Source: CAD feature listing. Evaluate the final solid. Frame: model axes, mm. Face numbers are marked on the shaded views. A direction names the side the tool comes from. Coordinates: 2 decimals unless noted, no trailing zeros. Write each loop counter-clockwise with the first axis right and the second up, starting at its lowest first coordinate (ties: lowest second). Pieces come first, ordered by that corner, then holes. Notation, with made-up numbers: M 15,13.5 L 50,13.5 A12 ccw 50,21.5 Z; hole C 45,78 d4. An arc over 180 degrees is marked long. One line per item, written item: value. Start each with the question number.
Item 1: Cut plane A-A, the plane z = 50. Output: boundary loops of the cut face in (x, y).
Item 2: Ray query, L1, parallel to Y at x = -24.85, z = 28.5; L2, parallel to X at y = 27, z = 50; L3, parallel to Z at x = 24, y = -10. Return the intervals inside material, ascending. Write a range as from..to.
Item 3: Cut plane B-B, the plane y = -23. Output: boundary loops of the cut face in (x, z).
Item 4: Set-up query: the marked faces 5, 6 and 7. Return all of +Z, -Z, +X, -X, +Y, -Y with unobstructed straight access to the full face (end or side cutting, diameter ignored); none if empty.
Item 5: Cut plane C-C, the plane z = 23. Output: boundary loops of the cut face in (x, y).
Item 6: Pin query (flat end, axial travel): P1, Ø3, axis at x = -16.5, z = 50.5, coming from the -Y side; P2, Ø4, axis at x = -24.85, y = 5, coming from the +Z side; P3, Ø3, axis at x = 25.5, y = -6, coming from the +Z side. Return the tip coordinate at first contact, or that it passes through.
Item 7: Mould query, pull axis Z, two halves, no side actions, for the marked faces 1, 2, 3 and 4. Classes: released by +Z, released by -Z, zero draft, split by the parting line, or undercut.
Item 8: Cut plane D-D, the plane x = 1. Output: boundary loops of the cut face in (y, z).
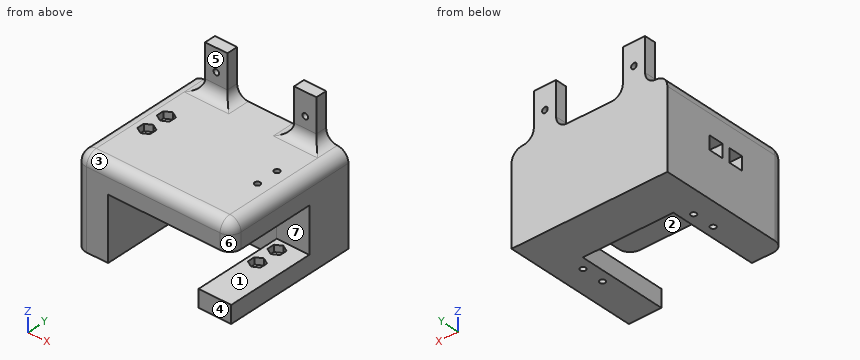
```python
from build123d import *

# Parameters (mm, degrees)
SKETCH_2_W           = 70
SKETCH_2_H           = 60
EXTRUDE_2_DEPTH      = 40
SKETCH_3_W           = 40.7
SKETCH_3_H           = 20.5
CUT_EXTRUDE_1_DEPTH  = 28
SKETCH_4_W           = 14.65
SKETCH_4_H           = 20.5
EXTRUDE_3_DEPTH      = 28
SKETCH_8_W           = 10
SKETCH_8_H           = 5
EXTRUDE_5_DEPTH      = 60
SKETCH_15_W          = 40.7
SKETCH_15_H          = 40.25
CUT_EXTRUDE_6_DEPTH  = 28
SKETCH_16_W          = 14.65
SKETCH_16_H          = 20.204149113
CUT_EXTRUDE_7_DEPTH  = 40
M3X0_5_1_D           = 2.5
FILLET_1_R           = 5
FILLET_2_R           = 5
FILLET_3_R           = 5
M3X0_5_2_D           = 2.5
CUT_EXTRUDE_8_DEPTH  = 3
CUT_EXTRUDE_9_DEPTH  = 3
CUT_EXTRUDE_10_DEPTH = 6


# Some blends are built 0.0001 mm under size
with BuildPart() as part:
    # ｽｹｯﾁ2 → ﾎﾞｽ - 押し出し2 (new body)
    with BuildSketch(Plane.XY):
        Rectangle(SKETCH_2_W, SKETCH_2_H)
    extrude(amount=EXTRUDE_2_DEPTH)

    # ｽｹｯﾁ3 → ｶｯﾄ - 押し出し1 (cut)
    with BuildSketch(Plane.XY):
        Rectangle(SKETCH_3_W, SKETCH_3_H)
    extrude(amount=CUT_EXTRUDE_1_DEPTH, mode=Mode.SUBTRACT)

    # ｽｹｯﾁ4 → ﾎﾞｽ - 押し出し3 (add)
    with BuildSketch(Plane.XY):
        with Locations((27.675, 0)):
            Rectangle(SKETCH_4_W, SKETCH_4_H)
    extrude(amount=EXTRUDE_3_DEPTH)

    # ｽｹｯﾁ8 → ﾎﾞｽ - 押し出し5 (add)
    with BuildSketch(Plane.XY):
        with Locations((-20, 27.5)):
            Rectangle(SKETCH_8_W, SKETCH_8_H)
        with Locations((20, 27.5)):
            Rectangle(SKETCH_8_W, SKETCH_8_H)
    extrude(amount=EXTRUDE_5_DEPTH)

    # ｽｹｯﾁ15 → ｶｯﾄ - 押し出し6 (cut)
    with BuildSketch(Plane.XY):
        with Locations((0, -9.875)):
            Rectangle(SKETCH_15_W, SKETCH_15_H)
    extrude(amount=CUT_EXTRUDE_6_DEPTH, mode=Mode.SUBTRACT)

    # ｽｹｯﾁ16 → ｶｯﾄ - 押し出し7 (cut)
    with BuildSketch(Plane(origin=(0, -30, 0), x_dir=(-1, 0, 0), z_dir=(0, -1, 0))):
        with Locations((-27.675, -17.897925444)):
            Rectangle(SKETCH_16_W, SKETCH_16_H)
    extrude(amount=-CUT_EXTRUDE_7_DEPTH, mode=Mode.SUBTRACT)

    # M3x0.5 ねじ穴1 (through all)
    with Locations(Plane(origin=(0, 30, 0), x_dir=(1, 0, 0), z_dir=(0, 1, 0))):
        with Locations((-20, -50), (20, -50)):
            Hole(M3X0_5_1_D / 2)

    # ﾌｨﾚｯﾄ1
    fillet_1_edges = [part.edges().sort_by_distance(p)[0] for p in [
        (-15, 27.5, 40),
        (-20, 25, 40),
        (-25, 27.5, 40),
        (20, 25, 40),
        (15, 27.5, 40),
        (25, 27.5, 40),
    ]]
    fillet(fillet_1_edges, radius=FILLET_1_R)

    # ﾌｨﾚｯﾄ2
    fillet_2_edges = [part.edges().sort_by_distance(p)[0] for p in [
        (35, 0, 40),
        (35, -30, 34),
        (0, -30, 40),
        (-35, 0, 40),
    ]]
    fillet(fillet_2_edges, radius=FILLET_2_R - 0.0001)  # a hair under: the kernel refuses the full size

    # ﾌｨﾚｯﾄ3
    # the kernel refuses this fillet: 5 mm, written as the material it takes off along each edge
    with BuildSketch(Plane(origin=(-30, -25, 40), x_dir=(-1, 0, 0), z_dir=(0, 1, 0))) as fillet_3_piece_1:
        with BuildLine():
            CenterArc((0.0001, -4.9999), 4.9999, 0, 90)
            Line((5, -4.9999), (5, 0))
            Line((5, 0), (0.0001, 0))
        make_face()
    revolve(axis=Axis((-30, -25, 40), (0, 0, 1)), revolution_arc=90, mode=Mode.SUBTRACT)
    with BuildSketch(Plane(origin=(-35, -30, -12.5), x_dir=(0, 1, 0), z_dir=(0, 0, 1))) as fillet_3_piece_2:
        with BuildLine():
            CenterArc((FILLET_3_R, -FILLET_3_R), FILLET_3_R, 90, 90)
            Line((0, -FILLET_3_R), (0, 0))
            Line((0, 0), (FILLET_3_R, 0))
        make_face()
    extrude(amount=52.5, mode=Mode.SUBTRACT)

    # M3x0.5 ねじ穴2 (through all)
    with Locations(Plane(origin=(0, 0, 0), x_dir=(-1, 0, 0), z_dir=(0, 0, -1))):
        with Locations((24.85, 5), (24.85, -5)):
            m3x0_5_2 = Hole(M3X0_5_2_D / 2)

    # ﾐﾗｰ1: M3x0.5 ねじ穴2 across plane
    add(m3x0_5_2.mirror(Plane(origin=(0, 0, 0), x_dir=(0, 0, 1), z_dir=(1, 0, 0))), mode=Mode.SUBTRACT)

    # ｽｹｯﾁ17 → ｶｯﾄ - 押し出し8 (cut)
    with BuildSketch(Plane.XY.offset(40)):
        Polygon((-24.85, 8.290896534), (-27.7, 6.645448267), (-27.7, 3.354551733), (-24.85, 1.709103466), (-22, 3.354551733), (-22, 6.645448267), align=None)
        Polygon((-22, -6.645448267), (-22, -3.354551733), (-24.85, -1.709103466), (-27.7, -3.354551733), (-27.7, -6.645448267), (-24.85, -8.290896534), align=None)
    extrude(amount=-CUT_EXTRUDE_8_DEPTH, mode=Mode.SUBTRACT)

    # ｽｹｯﾁ18 → ｶｯﾄ - 押し出し9 (cut)
    with BuildSketch(Plane.XY.offset(7.795850887)):
        Polygon((27.7, 3.354551733), (27.7, 6.645448267), (24.85, 8.290896534), (22, 6.645448267), (22, 3.354551733), (24.85, 1.709103466), align=None)
        Polygon((27.7, -6.645448267), (27.7, -3.354551733), (24.85, -1.709103466), (22, -3.354551733), (22, -6.645448267), (24.85, -8.290896534), align=None)
    extrude(amount=-CUT_EXTRUDE_9_DEPTH, mode=Mode.SUBTRACT)

    # ｽｹｯﾁ19 → ｶｯﾄ - 押し出し10 (cut)
    with BuildSketch(Plane(origin=(0, 0, 20), x_dir=(-1, 0, 0), z_dir=(0, 0, -1))):
        Polygon((35, 1.709103466), (35, 8.290896534), (24.85, 8.290896534), (27.7, 6.645448267), (27.7, 3.354551733), (24.85, 1.709103466), align=None)
        Polygon((22, 6.645448267), (22, 3.354551733), (24.85, 1.709103466), (27.7, 3.354551733), (27.7, 6.645448267), (24.85, 8.290896534), align=None)
        Polygon((22, -6.645448267), (24.85, -8.290896534), (27.7, -6.645448267), (27.7, -3.354551733), (24.85, -1.709103466), (22, -3.354551733), align=None)
        Polygon((35, -8.290896534), (24.85, -8.290896534), (27.7, -6.645448267), (27.7, -3.354551733), (24.85, -1.709103466), (35, -1.709103466), align=None)
    extrude(amount=-CUT_EXTRUDE_10_DEPTH, mode=Mode.SUBTRACT)


solid = part.part
```
From the geometry:
1. outline: M -25,25 L -21.25,25 L -21.25,30 L -25,30 Z; M -18.75,25 L -15,25 L -15,30 L -18.75,30 Z; M 15,25 L 18.75,25 L 18.75,30 L 15,30 Z; M 21.25,25 L 25,25 L 25,30 L 21.25,30 Z
2. L1: y = -30..-6.25, -3.75..3.75, 6.25..30
2. L2: x = -25..-21.25, -18.75..-15, 15..18.75, 21.25..25
2. L3: z = 0..7.8, 28..40
3. outline: M -35,0 L -20.35,0 L -20.35,28 L 35,28 L 35,35 A5 ccw 30,40 L -30,40 A5 ccw -35,35 Z; M 20.35,0 L 35,0 L 35,7.8 L 20.35,7.8 Z
4. face 5: +Z, +X, -X, -Y
4. face 6: +Z, +X, -Y
4. face 7: +X, -Y
5. outline: M -35,-25 A5 ccw -30,-30 L -20.35,-30 L -20.35,10.25 L 20.35,10.25 L 20.35,10 L 35,10 L 35,30 L -35,30 L -35,8.29 L -24.85,8.29 L -22,6.65 L -22,3.35 L -24.85,1.71 L -35,1.71 L -35,-1.71 L -24.85,-1.71 L -22,-3.35 L -22,-6.65 L -24.85,-8.29 L -35,-8.29 Z
6. P1: stops at y = 25
6. P2: stops at z = 37
6. P3: stops at z = 40
7. face 1: undercut
7. face 2: undercut
7. face 3: released by +Z
7. face 4: zero draft
8. outline: M -30,28 L 10.25,28 L 10.25,0 L 30,0 L 30,40 L -25,40 A5 ccw -30,35 Z
